Autodesk Inventor part; units mm, degrees
ref_plane "Start plane" through (0, 0, 0) normal (0, 0, 1) x (1, 0, 0)
ref_plane "End plane" through (0, 0, 730) normal (0, 0, 1) x (1, 0, 0)
ref_plane "Work Plane4" through (0, 0, 365) normal (-1, 0, 0) x (0, 0, 1)
ref_plane "Start plane" through (0, 0, 0) normal (0, 0, 1) x (1, 0, 0)
ref_plane "End plane" through (0, 0, 730) normal (0, 0, 1) x (1, 0, 0)
sketch "Sketch" plane through (0, 0, 0) normal (0, 0, 1) x (1, 0, 0)
  line L0 (-17.5, -14.3) -> (-17.5, 14.3)
  line L1 (-14.3, 17.5) -> (14.3, 17.5)
  line L2 (17.5, 14.3) -> (17.5, -14.3)
  line L3 (14.3, -17.5) -> (-14.3, -17.5)
  arc A0 (-17.5, -14.3) -> (-14.3, -17.5) centre (-14.3, -14.3) ccw
  arc A1 (-14.3, 17.5) -> (-17.5, 14.3) centre (-14.3, 14.3) ccw
  arc A2 (17.5, 14.3) -> (14.3, 17.5) centre (14.3, 14.3) ccw
  arc A3 (14.3, -17.5) -> (17.5, -14.3) centre (14.3, -14.3) ccw
  arc A4 (-14.3, 15.9) -> (-15.9, 14.3) centre (-14.3, 14.3) ccw
  line L4 (-14.3, 15.9) -> (14.3, 15.9)
  arc A5 (15.9, 14.3) -> (14.3, 15.9) centre (14.3, 14.3) ccw
  line L5 (15.9, 14.3) -> (15.9, -14.3)
  arc A6 (14.3, -15.9) -> (15.9, -14.3) centre (14.3, -14.3) ccw
  line L6 (14.3, -15.9) -> (-14.3, -15.9)
  arc A7 (-15.9, -14.3) -> (-14.3, -15.9) centre (-14.3, -14.3) ccw
  line L7 (-15.9, -14.3) -> (-15.9, 14.3)
  line L8 (0, 25.4278) -> (0, -25.4278) construction
  line L9 (-25.4278, 0) -> (25.4278, 0) construction
  dimension "d7" = 3.2
  dimension "d10" = 35
  dimension "d11" = 35
  dimension "d12" = 1.6
  dimension "d15" = 17.5
  dimension "d16" = 17.5
extrude "Body" add sketch "Sketch" along normal up to surface (730 mm away) from surface at 0
sketch "Sketch3" plane through (0, 0, 0) normal (0, 0, 1) x (1, 0, 0)
  line L0 (0, 0) -> (10, 0)
ref_plane "Work Plane3" through (0, 0, 0) normal (0, -1, 0) x (1, 0, 0)
sketch "Sketch4" plane through (0, 0, 0) normal (0, -1, 0) x (1, 0, 0)
  line L0 (-2, 0) -> (12, 0)
  line L1 (-2, 730) -> (12, 730)
  dimension "d18" = 730
ref_plane "Work Plane4" through (0, 0, 365) normal (-1, 0, 0) x (0, 0, 1)
ref_plane "Work Plane5" through (-430, 0, 365) normal (-1, 0, 0) x (0, 0, 1)
ref_plane "Work Plane6" through (-215, 0, 365) normal (-1, 0, 0) x (0, 0, 1)
sketch "Sketch5" plane through (-215, 0, 365) normal (-1, 0, 0) x (0, 0, 1)
  arc A0 (-17.5, -14.3) -> (-14.3, -17.5) centre (-14.3, -14.3) ccw
  line L0 (-17.5, -14.3) -> (-17.5, 14.3)
  arc A1 (-14.3, 17.5) -> (-17.5, 14.3) centre (-14.3, 14.3) ccw
  line L1 (-14.3, 17.5) -> (14.3, 17.5)
  arc A2 (17.5, 14.3) -> (14.3, 17.5) centre (14.3, 14.3) ccw
  line L2 (17.5, 14.3) -> (17.5, -14.3)
  arc A3 (14.3, -17.5) -> (17.5, -14.3) centre (14.3, -14.3) ccw
  line L3 (14.3, -17.5) -> (-14.3, -17.5)
  arc A4 (-14.3, 15.9) -> (-15.9, 14.3) centre (-14.3, 14.3) ccw
  line L4 (-14.3, 15.9) -> (14.3, 15.9)
  arc A5 (15.9, 14.3) -> (14.3, 15.9) centre (14.3, 14.3) ccw
  line L5 (15.9, 14.3) -> (15.9, -14.3)
  arc A6 (14.3, -15.9) -> (15.9, -14.3) centre (14.3, -14.3) ccw
  line L6 (14.3, -15.9) -> (-14.3, -15.9)
  arc A7 (-15.9, -14.3) -> (-14.3, -15.9) centre (-14.3, -14.3) ccw
  line L7 (-15.9, -14.3) -> (-15.9, 14.3)
extrude "Extrusion2" cut sketch "Sketch5" along normal up to surface (430 mm away) from surface at -215 contours L0 A1 L1 A2 L2 A3 L3 A0 | L4 A5 L5 A6 L6 A7 L7 A4
equation "\"d7\" = G_IR"
equation "\"d10\" = G_H"
equation "\"d11\" = G_W"
equation "\"d12\" = G_T"
equation "\"d15\" = 0.5 * d10"
equation "\"d16\" = 0.5 * d11"
equation "\"d3\" = G_L"
equation "\"G_W\" = 35"
equation "\"G_H\" = 35"
equation "\"G_T\" = 1.6"
equation "\"G_IR\" = 3.2"
equation "\"G_L\" = d18"
equation "\"G_OFFSET_START\" = 0"
equation "\"G_OFFSET_END\" = 0"
properties part number "AS 1163 - C350L0 35x35x1.6 SHS - 730" material "Steel, Mild"
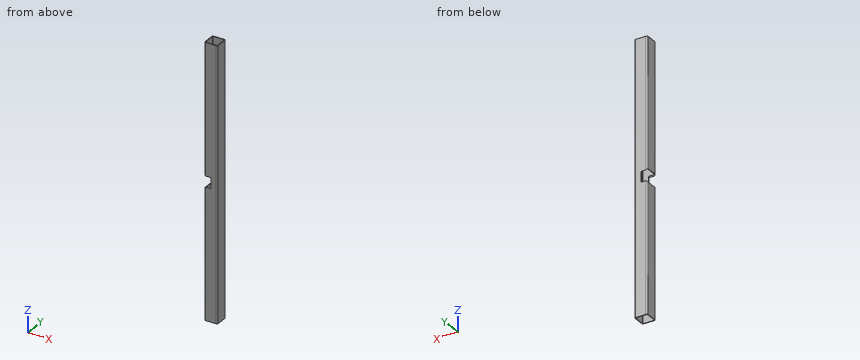
The model under review builds one solid part; all positions refer to its coordinate system, in mm. Round coordinates to 2 decimals unless told otherwise and drop trailing zeros. Loops run counter-clockwise (first coordinate to the right, second up) from the corner with the lowest first, then second, coordinate; pieces in that order, holes last. Notation, with made-up numbers: M 26,31 L 68,31 A36 ccw 68,68 Z; hole C 22.5,-34 d7. An arc over 180 degrees is marked long. Write item = value, one per line.
Item 1: Take a section at B-B on z = 673. Write out the cut boundary in (x, y), then the cut area to 3 significant figures.
Return value:
outline = M -17.5,-14.3 A3.2 ccw -14.3,-17.5 L 14.3,-17.5 A3.2 ccw 17.5,-14.3 L 17.5,14.3 A3.2 ccw 14.3,17.5 L -14.3,17.5 A3.2 ccw -17.5,14.3 Z; hole M -15.9,-14.3 A1.6 ccw -14.3,-15.9 L 14.3,-15.9 A1.6 ccw 15.9,-14.3 L 15.9,14.3 A1.6 ccw 14.3,15.9 L -14.3,15.9 A1.6 ccw -15.9,14.3 Z
area = 207 mm2
Item 2: Take a section at C-C on y = 2. Write out the cut boundary in (x, z).
Return value:
outline = M -17.5,0 L -15.9,0 L -15.9,347.5 L -17.5,347.5 Z; M -17.5,382.5 L -15.9,382.5 L -15.9,730 L -17.5,730 Z; M 15.9,0 L 17.5,0 L 17.5,730 L 15.9,730 Z
Item 3: Take a section at A-A on x = -9. Write out the cut boundary in (y, z).
Return value:
outline = M -17.5,0 L -15.9,0 L -15.9,347.93 A3.2 cw -17.5,350.7 Z; M -17.5,379.3 A3.2 cw -15.9,382.07 L -15.9,730 L -17.5,730 Z; M 15.9,0 L 17.5,0 L 17.5,350.7 A3.2 cw 15.9,347.93 Z; M 15.9,382.07 A3.2 cw 17.5,379.3 L 17.5,730 L 15.9,730 Z
Item 4: Insertion check: P1, Ø1.3, axis at y = -17, z = 366, coming from the -X side; P2, Ø10, axis at x = 8.5, y = 10, coming from the -Z side. Each pin has a flat end and moves straight along its axis. Give the tip position at first contact, or say it passes through.
Return value:
P1 = 0
P2 = through
Item 5: For line 1 (Y direction, x = -11, z = 35); line 2 (X direction, y = 15, z = 204.5), list the stretches that pass through material, from the lowest coordinate up. Write a range as [from, to].
Return value:
line_1 = [-17.5, -15.9], [15.9, 17.5]
line_2 = [-17.42, -15.74], [15.74, 17.42]
